Verification items for the finished model (mm, model axes). Coordinates: 2 decimals unless noted, no trailing zeros. Loops run counter-clockwise (first coordinate to the right, second up) from the corner with the lowest first, then second, coordinate; pieces in that order, holes last. Notation, with made-up numbers: (-1, 80) - (15, 80) arc R23 ccw to (15, 99) - close; hole circle Ø4 at (58, 70.25). An arc over 180 degrees is marked (long way). Answer as CSV lines item,"result". Start each with the question number.
1. Gauge pin test, flat end, axial feed: P1, Ø0.6, axis at y = 4, z = 6.5, coming from the +X side. Record the tip position at first contact, or that the pin passes through.
2. Cross-section at B-B (z = 0.5). Enter the section's corners in (x, y).
3. Material ranges on line 1 (X direction, y = 3.65, z = 0); line 2 (Z direction, x = -7, y = 1.6); line 3 (Z direction, x = 10.5, y = 3.75), recorded low to high. Write a range as [from, to].
4. Cross-section at A-A (x = -2). Enter the section's corners in (y, z).
5. Cross-section at C-C (y = 2). Enter the section's corners in (x, z).
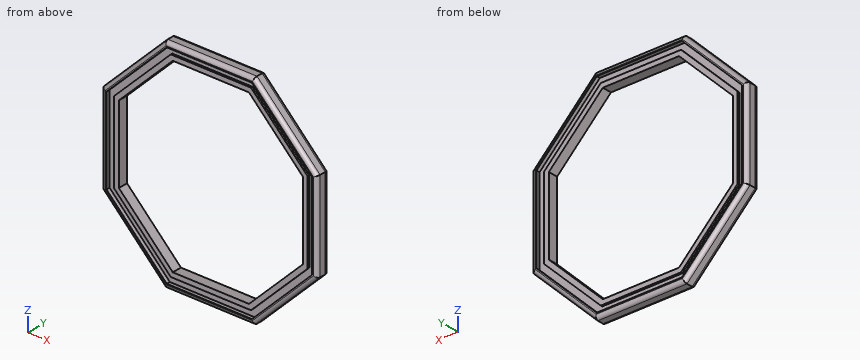
Autodesk Inventor part; units mm, degrees
ref_plane "작업 평면3" through (0, 2.2, 0) normal (0, -1, 0) x (1, 0, 0)
ref_plane "YZ Plane" through (0, 0, 0) normal (1, 0, 0) x (0, 1, 0)
ref_plane "XZ Plane" through (0, 0, 0) normal (0, 1, 0) x (-1, 0, 0)
sketch "스케치1" plane through (0, 0, 0) normal (0, 1, 0) x (-1, 0, 0)
  line L0 (-32.5919, 13.5) -> (-13.5, 32.5919)
  line L1 (-13.5, 32.5919) -> (13.5, 32.5919)
  line L2 (13.5, 32.5919) -> (32.5919, 13.5)
  line L3 (32.5919, 13.5) -> (32.5919, -13.5)
  line L4 (32.5919, -13.5) -> (13.5, -32.5919)
  line L5 (13.5, -32.5919) -> (-13.5, -32.5919)
  line L6 (-13.5, -32.5919) -> (-32.5919, -13.5)
  line L7 (-32.5919, -13.5) -> (-32.5919, 13.5)
  line L8 (35.7919, 14.8255) -> (35.7919, -14.8255)
  line L9 (35.7919, -14.8255) -> (14.8255, -35.7919)
  line L10 (14.8255, -35.7919) -> (-14.8255, -35.7919)
  line L11 (-14.8255, -35.7919) -> (-35.7919, -14.8255)
  line L12 (-35.7919, -14.8255) -> (-35.7919, 14.8255)
  line L13 (-35.7919, 14.8255) -> (-14.8255, 35.7919)
  line L14 (-14.8255, 35.7919) -> (14.8255, 35.7919)
  line L15 (14.8255, 35.7919) -> (35.7919, 14.8255)
  point P0 (0, 0)
  point P1 (0, 0)
  point P2 (0, 0)
  dimension "d0" = 27
  dimension "d1" = 3.2
extrude "돌출1" add sketch "스케치1" along normal blind 4.4 contours L0 L1 L2 L3 L4 L5 L6 L7 | L8 L9 L10 L11 L12 L13 L14 L15
sketch "스케치3" plane through (0, 0, 0) normal (0, -1, 0) x (1, 0, 0)
  line L0 (-13.3343, 32.1919) -> (13.3343, 32.1919)
  line L1 (13.3343, 32.1919) -> (32.1919, 13.3343)
  line L2 (32.1919, 13.3343) -> (32.1919, -13.3343)
  line L3 (32.1919, -13.3343) -> (13.3343, -32.1919)
  line L4 (13.3343, -32.1919) -> (-13.3343, -32.1919)
  line L5 (-13.3343, -32.1919) -> (-32.1919, -13.3343)
  line L6 (-32.1919, -13.3343) -> (-32.1919, 13.3343)
  line L7 (-32.1919, 13.3343) -> (-13.3343, 32.1919)
  line L8 (-14.1627, 34.1919) -> (14.1627, 34.1919)
  line L9 (14.1627, 34.1919) -> (34.1919, 14.1627)
  line L10 (34.1919, 14.1627) -> (34.1919, -14.1627)
  line L11 (34.1919, -14.1627) -> (14.1627, -34.1919)
  line L12 (14.1627, -34.1919) -> (-14.1627, -34.1919)
  line L13 (-14.1627, -34.1919) -> (-34.1919, -14.1627)
  line L14 (-34.1919, -14.1627) -> (-34.1919, 14.1627)
  line L15 (-34.1919, 14.1627) -> (-14.1627, 34.1919)
  line L16 (-14.8255, 35.7919) -> (14.8255, 35.7919)
  point P0 (0, 0)
  point P1 (0, 0)
  point P2 (0, 0)
  point P3 (0, 0)
  dimension "d9" = 2
  dimension "d144" = 1.6
extrude "돌출3" cut sketch "스케치3" against normal blind 1.2
sketch "스케치14" plane through (0, 0, 0) normal (0, -1, 0) x (1, 0, 0)
  line L0 (32.1919, 13.3343) -> (13.3343, 32.1919)
  line L1 (13.3343, 32.1919) -> (-13.3343, 32.1919)
  line L2 (-13.3343, 32.1919) -> (-32.1919, 13.3343)
  line L3 (-32.1919, 13.3343) -> (-32.1919, -13.3343)
  line L4 (-32.1919, -13.3343) -> (-13.3343, -32.1919)
  line L5 (-13.3343, -32.1919) -> (13.3343, -32.1919)
  line L6 (13.3343, -32.1919) -> (32.1919, -13.3343)
  line L7 (32.1919, -13.3343) -> (32.1919, 13.3343)
  point P0 (0, 0)
extrude "돌출16" cut sketch "스케치14" against normal blind 0.6
sketch "스케치15" plane through (0, 0.6, 0) normal (0, -1, 0) x (1, 0, 0)
  line L0 (-12.6716, 30.5919) -> (12.6716, 30.5919)
  line L1 (12.6716, 30.5919) -> (30.5919, 12.6716)
  line L2 (30.5919, 12.6716) -> (30.5919, -12.6716)
  line L3 (30.5919, -12.6716) -> (12.6716, -30.5919)
  line L4 (12.6716, -30.5919) -> (-12.6716, -30.5919)
  line L5 (-12.6716, -30.5919) -> (-30.5919, -12.6716)
  line L6 (-30.5919, -12.6716) -> (-30.5919, 12.6716)
  line L7 (-30.5919, 12.6716) -> (-12.6716, 30.5919)
  line L8 (-13.3343, 32.1919) -> (13.3343, 32.1919)
  point P0 (0, 0)
  point P1 (0, 0)
  dimension "d140" = 1.6
extrude "돌출17" cut sketch "스케치15" against normal up to surface (3.8 mm away)
ref_plane "작업 평면3" through (0, 2.2, 0) normal (0, -1, 0) x (1, 0, 0)
mirror "미러6" about plane through (0, 2.2, 0) normal (0, -1, 0) of "돌출3", "돌출16"
fillet "모깎기2" radius 1.2 16 edges at (0, 0, 35.7919) (-25.3087, 0, 25.3087) (-35.7919, 0, 0) (-25.3087, 0, -25.3087) (0, 0, -35.7919) (25.3087, 0, -25.3087) (35.7919, 0, 0) (25.3087, 0, 25.3087) (-25.3087, 4.4, 25.3087) (-35.7919, 4.4, 0) (-25.3087, 4.4, -25.3087) (0, 4.4, -35.7919) (25.3087, 4.4, -25.3087) (35.7919, 4.4, 0) (25.3087, 4.4, 25.3087) (0, 4.4, 35.7919)
properties part number "OV-PAM_ring_2"
Values follow:
1,P1,"stops at x = 35.68"
2,outline,"(-35.79, 1.2) arc R1.2 ccw to (-34.59, 0) - (-34.19, 0) - (-34.19, 1.2) - (-32.19, 1.2) - (-32.19, 0.6) - (-30.59, 0.6) - (-30.59, 3.8) - (-32.19, 3.8) - (-32.19, 3.2) - (-34.19, 3.2) - (-34.19, 4.4) - (-34.59, 4.4) arc R1.2 ccw to (-35.79, 3.2) - close; (30.59, 0.6) - (32.19, 0.6) - (32.19, 1.2) - (34.19, 1.2) - (34.19, 0) - (34.59, 0) arc R1.2 ccw to (35.79, 1.2) - (35.79, 3.2) arc R1.2 ccw to (34.59, 4.4) - (34.19, 4.4) - (34.19, 3.2) - (32.19, 3.2) - (32.19, 3.8) - (30.59, 3.8) - close"
3,line 1,"x = [-35.7, -34.19], [-32.19, -30.59], [30.59, 32.19], [34.19, 35.7]"
3,line 2,"z = [-35.79, -30.59], [30.59, 35.79]"
3,line 3,"z = [-35.66, -34.19], [-32.19, -30.59], [30.59, 32.19], [34.19, 35.66]"
4,outline,"(0, -34.59) arc R1.2 ccw to (1.2, -35.79) - (3.2, -35.79) arc R1.2 ccw to (4.4, -34.59) - (4.4, -34.19) - (3.2, -34.19) - (3.2, -32.19) - (3.8, -32.19) - (3.8, -30.59) - (0.6, -30.59) - (0.6, -32.19) - (1.2, -32.19) - (1.2, -34.19) - (0, -34.19) - close; (0, 34.19) - (1.2, 34.19) - (1.2, 32.19) - (0.6, 32.19) - (0.6, 30.59) - (3.8, 30.59) - (3.8, 32.19) - (3.2, 32.19) - (3.2, 34.19) - (4.4, 34.19) - (4.4, 34.59) arc R1.2 ccw to (3.2, 35.79) - (1.2, 35.79) arc R1.2 ccw to (0, 34.59) - close"
5,outline,"(-35.79, -14.83) - (-14.83, -35.79) - (14.83, -35.79) - (35.79, -14.83) - (35.79, 14.83) - (14.83, 35.79) - (-14.83, 35.79) - (-35.79, 14.83) - close; hole (-30.59, -12.67) - (-12.67, -30.59) - (12.67, -30.59) - (30.59, -12.67) - (30.59, 12.67) - (12.67, 30.59) - (-12.67, 30.59) - (-30.59, 12.67) - close"
